Work out the finished part from the listing and answer in its coordinate system (mm). Face numbers are marked on the shaded views. A direction names the side the tool comes from. Coordinates: 2 decimals unless noted, no trailing zeros. Loops run counter-clockwise (first coordinate to the right, second up) from the corner with the lowest first, then second, coordinate; pieces in that order, holes last. Notation, with made-up numbers: (23.5, -14.75) - (60.5, -14.75) arc R16 ccw to (60.5, 4.25) - close; hole circle Ø3 at (10, 59.25). An arc over 180 degrees is marked (long way). Write each question's results on one line, items separated by ' | '. Start each with the question number.
1. Which of the six approach directions +Z, -Z, +X, -X, +Y, -Y give full straight-line access (tool end or side, diameter ignored) to the marked faces 5, 6 and 7?
2. A cutting plane is placed at C-C on x = 0. Determine the outline of the cut face in (y, z).
3. A cutting plane is placed at A-A on y = 0. Determine the outline of the cut face in (x, z), then the cut area to 3 significant figures.
4. Each of these flat-tipped pins is pushed along its axis until it touches: P1, Ø5, axis at x = -7.5, y = 2, coming from the +Z side; P2, Ø5, axis at x = 9.5, z = -9.5, coming from the -Y side; P3, Ø9, axis at y = 28.5, z = -20.5, coming from the +X side; P4, Ø1.2, axis at x = 4, y = 22, coming from the -Z side. Where does it stop, or does it pass through?
5. Find the intervals of material crossed by line 1 along Y through (x, z) = (-15.5, 0.3); line 2 along Y through (x, z) = (-17.3, -15.75); line 3 along Y through (x, z) = (3, -14.5), in increasing order. Write a range as [from, to].
6. A cutting plane is placed at D-D on x = -15. Determine the outline of the cut face in (y, z).
7. A cutting plane is placed at B-B on z = -15.75. Determine the outline of the cut face in (x, y), then the cut area to 3 significant figures.
8. Determine the mould class of the marked faces 1, 2, 3 and 4 for opening direction Y: released by +Y, released by -Y, zero draft, split by the parting line, or undercut.
Autodesk Inventor part; units mm, degrees
ref_plane "Work Plane1" through (-21.15, -21.15, -31.5) normal (0, 0, -1) x (0, 1, 0)
ref_plane "YZ Plane" through (0, 0, 0) normal (1, 0, 0) x (0, 1, 0)
ref_plane "XZ Plane" through (0, 0, 0) normal (0, 1, 0) x (-1, 0, 0)
sketch "Sketch1" plane through (0, 0, 0) normal (0, 0, 1) x (1, 0, 0)
  line L0 (20.0607, 17.4322) -> (17.4322, 20.0607) construction
  arc A0 (17.4322, 20.0607) -> (16.3716, 20.5) centre (16.3716, 19) ccw construction
  line L1 (16.3716, 20.5) -> (-16.3716, 20.5) construction
  arc A1 (-16.3716, 20.5) -> (-17.4322, 20.0607) centre (-16.3716, 19) ccw construction
  line L2 (-17.4322, 20.0607) -> (-20.0607, 17.4322) construction
  arc A2 (-20.0607, 17.4322) -> (-20.5, 16.3716) centre (-19, 16.3716) ccw construction
  line L3 (-20.5, 16.3716) -> (-20.5, -16.3716) construction
  arc A3 (-20.5, -16.3716) -> (-20.0607, -17.4322) centre (-19, -16.3716) ccw construction
  line L4 (-20.0607, -17.4322) -> (-17.4322, -20.0607) construction
  arc A4 (-17.4322, -20.0607) -> (-16.3716, -20.5) centre (-16.3716, -19) ccw construction
  line L5 (-16.3716, -20.5) -> (16.3716, -20.5) construction
  arc A5 (16.3716, -20.5) -> (17.4322, -20.0607) centre (16.3716, -19) ccw construction
  line L6 (17.4322, -20.0607) -> (20.0607, -17.4322) construction
  arc A6 (20.0607, -17.4322) -> (20.5, -16.3716) centre (19, -16.3716) ccw construction
  line L7 (20.5, -16.3716) -> (20.5, 16.3716) construction
  arc A7 (20.5, 16.3716) -> (20.0607, 17.4322) centre (19, 16.3716) ccw construction
  circle A8 centre (0, 0) radius 16.5 construction
  circle A9 centre (15.5, 15.5) radius 1.55 construction
  circle A10 centre (15.5, -15.5) radius 1.55 construction
  circle A11 centre (-15.5, -15.5) radius 1.55 construction
  circle A12 centre (-15.5, 15.5) radius 1.55 construction
  line L8 (0, 0) -> (-20.3858, 0) construction
  line L9 (-20.3858, 0) -> (-20.3858, -20.3858) construction
  line L10 (-20.3858, -20.3858) -> (0, -20.3858) construction
  line L11 (0, -20.3858) -> (0, 0) construction
  line L12 (0, 0) -> (-20.3858, 0) construction
  line L13 (-20.3858, 0) -> (-20.3858, 20.3858) construction
  line L14 (-20.3858, 20.3858) -> (0, 20.3858) construction
  line L15 (0, 20.3858) -> (0, 0) construction
  line L16 (0, 0) -> (20.3858, 0) construction
  line L17 (20.3858, 0) -> (20.3858, 20.3858) construction
  line L18 (20.3858, 20.3858) -> (0, 20.3858) construction
  line L19 (0, 20.3858) -> (0, 0) construction
  line L20 (0, 0) -> (20.3858, 0) construction
  line L21 (20.3858, 0) -> (20.3858, -20.3858) construction
  line L22 (20.3858, -20.3858) -> (0, -20.3858) construction
  line L23 (0, -20.3858) -> (0, 0) construction
  line L24 (-20.3858, -20.3858) -> (20.3858, -20.3858)
  line L25 (20.3858, -20.3858) -> (20.3858, 20.3858)
  line L26 (20.3858, 20.3858) -> (-20.3858, 20.3858)
  line L27 (-20.3858, 20.3858) -> (-20.3858, -20.3858)
  line L28 (-21.15, -107.4) -> (-21.15, 107.4)
  line L29 (-21.15, 22.8858) -> (22.8858, 22.8858)
  line L30 (22.8858, 22.8858) -> (22.8858, -22.8858)
  line L31 (22.8858, -22.8858) -> (-21.15, -22.8858)
  point P0 (0, 0)
  dimension "d0" = 2.5
ref_plane "Work Plane1" through (-21.15, -21.15, -31.5) normal (0, 0, -1) x (0, 1, 0)
extrude "Extrusion1" add sketch "Sketch1" against normal up to surface (31.5 mm away)
ref_plane "Work Plane2" through (-21.15, -10, -125) normal (1, 0, 0) x (0, 0, 1)
sketch "Sketch2" plane through (-21.15, -10, -125) normal (1, 0, 0) x (0, 0, 1)
  line L0 (125, 12.8858) -> (125, -32.8858)
  line L1 (93.5, 12.8858) -> (93.5, -32.8858)
  line L2 (125, -32.8858) -> (93.5, -32.8858)
  line L3 (125, 12.8858) -> (125, -32.8858)
  line L4 (125, 12.8858) -> (93.5, 12.8858)
  line L5 (125, -10) -> (93.5, -10) construction
  line L6 (109.25, 12.8858) -> (109.25, -32.8858) construction
  line L7 (109.25, -32.8858) -> (119.25, -32.8858) construction
  line L8 (119.25, -32.8858) -> (119.25, -42.8858)
  line L9 (119.25, -42.8858) -> (109.25, -42.8858)
  line L10 (109.25, -42.8858) -> (109.25, -32.8858) construction
  line L11 (109.25, -42.8858) -> (99.25, -42.8858)
  line L12 (99.25, -42.8858) -> (99.25, -32.8858)
  line L13 (99.25, -32.8858) -> (109.25, -32.8858) construction
  line L14 (109.25, -32.8858) -> (109.25, -42.8858) construction
  line L15 (125, 12.8858) -> (93.5, 12.8858)
  line L16 (119.25, 12.8858) -> (119.25, 22.8858)
  line L17 (119.25, 22.8858) -> (109.25, 22.8858)
  line L18 (109.25, 22.8858) -> (99.25, 22.8858)
  line L19 (99.25, 22.8858) -> (99.25, 12.8858)
  dimension "d3" = 10
  dimension "d4" = 10
  dimension "d5" = 10
  dimension "d6" = 10
extrude "Extrusion2" add sketch "Sketch2" along normal blind 5 contours L4 L19 L18 L17 L16 | L8 L9 L11 L12 L2
sketch "Sketch3" plane through (0, 0, 0) normal (0, 0, 1) x (1, 0, 0)
  line L0 (22.8858, 22.8858) -> (-21.15, 22.8858)
  line L1 (-21.15, 22.8858) -> (-21.15, -22.8858)
  line L2 (22.8858, 22.8858) -> (-21.15, 22.8858)
  line L3 (-21.15, 22.8858) -> (-21.15, -22.8858)
  line L4 (-21.15, -22.8858) -> (22.8858, -22.8858)
  line L5 (22.8858, -22.8858) -> (22.8858, 22.8858)
  circle A0 centre (-15.5, 15.5) radius 1.25
  circle A1 centre (15.5, 15.5) radius 1.25
  circle A2 centre (-15.5, -15.5) radius 1.25
  circle A3 centre (15.5, -15.5) radius 1.25
  circle A4 centre (0, 0) radius 11
  point P0 (0, 0)
extrude "Extrusion3" add sketch "Sketch3" along normal blind 1
fillet "Fillet1" radius 2 10 edges at (-18.65, 22.8858, -25.75) (-18.65, 32.8858, -25.75) (-18.65, 32.8858, -5.75) (-18.65, 22.8858, -5.75) (-18.65, -22.8858, -25.75) (-18.65, -32.8858, -25.75) (-18.65, -32.8858, -5.75) (-18.65, -22.8858, -5.75) (-16.15, -22.8858, -15.75) (-16.15, 22.8858, -15.75)
sketch "Sketch4" plane through (-16.15, -10, -125) normal (1, 0, 0) x (0, 0, -1)
  arc A0 (-117.25, 42.8858) -> (-119.25, 40.8858) centre (-117.25, 40.8858) ccw
  line L0 (-119.25, 40.8858) -> (-119.25, 34.8858)
  line L1 (-99.25, 34.8858) -> (-119.25, 34.8858)
  line L2 (-99.25, 34.8858) -> (-99.25, 40.8858)
  arc A1 (-99.25, 40.8858) -> (-101.25, 42.8858) centre (-101.25, 40.8858) ccw
  line L3 (-101.25, 42.8858) -> (-117.25, 42.8858)
  arc A2 (-119.25, -20.8858) -> (-117.25, -22.8858) centre (-117.25, -20.8858) ccw
  line L4 (-117.25, -22.8858) -> (-101.25, -22.8858)
  arc A3 (-101.25, -22.8858) -> (-99.25, -20.8858) centre (-101.25, -20.8858) ccw
  line L5 (-99.25, -20.8858) -> (-99.25, -14.8858)
  line L6 (-119.25, -14.8858) -> (-99.25, -14.8858)
  line L7 (-119.25, -14.8858) -> (-119.25, -20.8858)
  circle A4 centre (-109.25, 38.7448) radius 2.5
  line L8 (-215.88, 9.0017) -> (215.88, 9.0017) construction
  line L9 (-126, 32.8858) -> (-126, -12.8858) construction
  line L10 (-126, 10) -> (-93.5, 10) construction
  line L11 (-93.5, 32.8858) -> (-93.5, -12.8858) construction
  circle A5 centre (-109.25, -18.7448) radius 2.5
  point P0 (-125, 10)
  dimension "d12" = 5
extrude "Extrusion4" cut sketch "Sketch4" against normal up to surface (5 mm away) contours A4 | A5
sketch "Sketch5" plane through (0, 0, 0) normal (0, 0, -1) x (-1, 0, 0)
  circle A0 centre (0, 0) radius 11
  circle A1 centre (0, 0) radius 11.5
  point P0 (0, 0)
  dimension "d15" = 0.5
extrude "Extrusion5" cut sketch "Sketch5" against normal up to surface (1 mm away) contours A0 | A1
sketch "Sketch6" plane through (22.8858, 22.8858, -31.5) normal (0, 0, -1) x (-1, 0, 0)
  line L0 (43.2716, -2.5) -> (2.5, -2.5)
  line L1 (43.2716, -43.2716) -> (43.2716, -2.5)
  line L2 (2.5, -43.2716) -> (43.2716, -43.2716)
  line L3 (2.5, -2.5) -> (2.5, -43.2716)
  line L4 (44.0358, 0) -> (44.0358, -45.7716)
  line L5 (0, 0) -> (44.0358, 0)
  line L6 (0, -45.7716) -> (0, 0)
  line L7 (44.0358, -45.7716) -> (0, -45.7716)
  line L8 (1.5, -44.2716) -> (44.2716, -44.2716)
  line L9 (44.2716, -44.2716) -> (44.2716, -1.5)
  line L10 (44.2716, -1.5) -> (1.5, -1.5)
  line L11 (1.5, -1.5) -> (1.5, -44.2716)
  line L12 (44.2716, -44.2716) -> (44.0358, -44.2716)
  line L13 (44.2716, -1.5) -> (44.0358, -1.5)
  point P0 (22.8858, -22.8858)
  dimension "d18" = 1
extrude "Extrusion6" cut sketch "Sketch6" against normal up to surface (31.5 mm away) contours L10 L9 L8 L4 | L4 L8 L11 L10
sketch "Sketch7" plane through (22.8858, -22.8858, -31.5) normal (1, 0, 0) x (0, 0, -1)
  line L0 (-10, 30.8858) -> (-10, 14.8858)
  line L1 (-10, 14.8858) -> (0, 14.8858)
  line L2 (0, 30.8858) -> (-10, 30.8858)
  line L3 (0, 1.5) -> (0, 44.2716)
  line L4 (-10, 30.8858) -> (0, 22.8858) construction
  line L5 (-10, 14.8858) -> (0, 22.8858) construction
  point P0 (-31.5, 22.8858)
  dimension "d21" = 16
extrude "Extrusion7" cut sketch "Sketch7" against normal up to surface (1.5 mm away)
sketch "Sketch8" plane through (-21.15, 22.8858, -31.5) normal (0, 1, 0) x (1, 0, 0)
  line L0 (29.2679, 0) -> (29.2679, -10)
  line L1 (29.2679, -10) -> (13.2679, -10)
  line L2 (13.2679, -10) -> (13.2679, 0)
  line L3 (42.5358, 0) -> (0, 0)
  line L4 (21.2679, 0) -> (29.2679, -10) construction
  line L5 (21.2679, 0) -> (13.2679, -10) construction
  point P0 (21.15, -31.5)
extrude "Extrusion8" cut sketch "Sketch8" against normal up to surface (45.7716 mm away)
sketch "Sketch9" plane through (0, 0, 1) normal (0, 0, 1) x (1, 0, 0)
  circle A0 centre (0, 0) radius 11.5
  line L0 (22.8858, 22.8858) -> (-21.15, 22.8858)
  line L1 (-21.15, 22.8858) -> (-21.15, -22.8858)
  line L2 (-21.15, -22.8858) -> (22.8858, -22.8858)
  line L3 (22.8858, -22.8858) -> (22.8858, 22.8858)
  circle A1 centre (15.5, -15.5) radius 1.25
  circle A2 centre (-15.5, -15.5) radius 1.25
  circle A3 centre (15.5, 15.5) radius 1.25
  circle A4 centre (-15.5, 15.5) radius 1.25
  circle A5 centre (-15.5, 15.5) radius 1.5
  circle A6 centre (15.5, 15.5) radius 1.5
  circle A7 centre (15.5, -15.5) radius 1.5
  circle A8 centre (-15.5, -15.5) radius 1.5
  point P0 (0, 0)
  dimension "d29" = 0.25
  dimension "d30" = 0.25
  dimension "d31" = 0.25
  dimension "d32" = 0.25
extrude "Extrusion9" cut sketch "Sketch9" against normal up to surface (1 mm away) contours A1 | A2 | A3 | A5 | A6 | A7 | A8
properties part number "Nema17WheelMotorMountoffset"
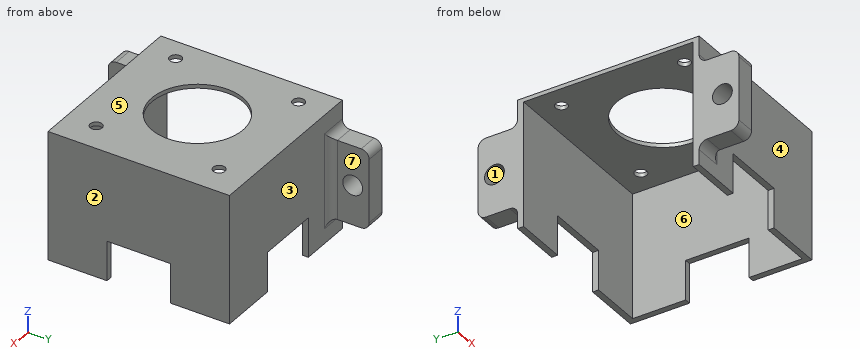
Values:
1) face 5: +Z, +X, -X, +Y, -Y | face 6: -Z, -X | face 7: +Z, -Z, +X, +Y
2) outline: (-22.89, -21.5) - (-21.39, -21.5) - (-21.39, 0) - (-11.5, 0) - (-11.5, 1) - (-22.89, 1) - close; (11.5, 0) - (21.39, 0) - (21.39, -21.5) - (22.89, -21.5) - (22.89, 1) - (11.5, 1) - close
3) outline: (-21.15, 0) - (-11.5, 0) - (-11.5, 1) - (-21.15, 1) - close; (11.5, 0) - (21.39, 0) - (21.39, -21.5) - (22.89, -21.5) - (22.89, 1) - (11.5, 1) - close | area: 53.3 mm^2
4) P1: through | P2: y = -22.89 | P3: x = -15.94 | P4: z = -21.5
5) line 1: [-22.89, -17], [-14, 14], [17, 22.89] | line 2: [-32.89, -31.24], [-26.24, -21.39], [21.39, 26.24], [31.24, 32.89] | line 3: [-22.89, -21.39], [21.39, 22.89]
6) outline: (-23.08, -26.9) arc R2 cw to (-22.89, -27.75) - (-22.89, -31.5) - (-21.39, -31.5) - (-21.39, 0) - (-16.91, 0) - (-16.91, 1) - (-22.89, 1) - (-22.89, -3.75) arc R2 cw to (-23.08, -4.6) - close; (-14.09, 0) - (14.09, 0) - (14.09, 1) - (-14.09, 1) - close; (16.91, 0) - (21.39, 0) - (21.39, -31.5) - (22.89, -31.5) - (22.89, -27.75) arc R2 cw to (23.08, -26.9) - (23.08, -4.6) arc R2 cw to (22.89, -3.75) - (22.89, 1) - (16.91, 1) - close
7) outline: (-21.15, -32.89) - (-16.15, -32.89) - (-16.15, -31.24) - (-21.15, -31.24) - close; (-21.15, -26.24) - (-16.15, -26.24) - (-16.15, -24.89) arc R2 cw to (-14.15, -22.89) - (22.89, -22.89) - (22.89, 22.89) - (-14.15, 22.89) arc R2 cw to (-16.15, 24.89) - (-16.15, 26.24) - (-21.15, 26.24) - (-21.15, 21.39) - (21.39, 21.39) - (21.39, -21.39) - (-21.15, -21.39) - close; (-21.15, 31.24) - (-16.15, 31.24) - (-16.15, 32.89) - (-21.15, 32.89) - close | area: 248 mm^2
8) face 1: undercut | face 2: zero draft | face 3: released by +Y | face 4: released by -Y
